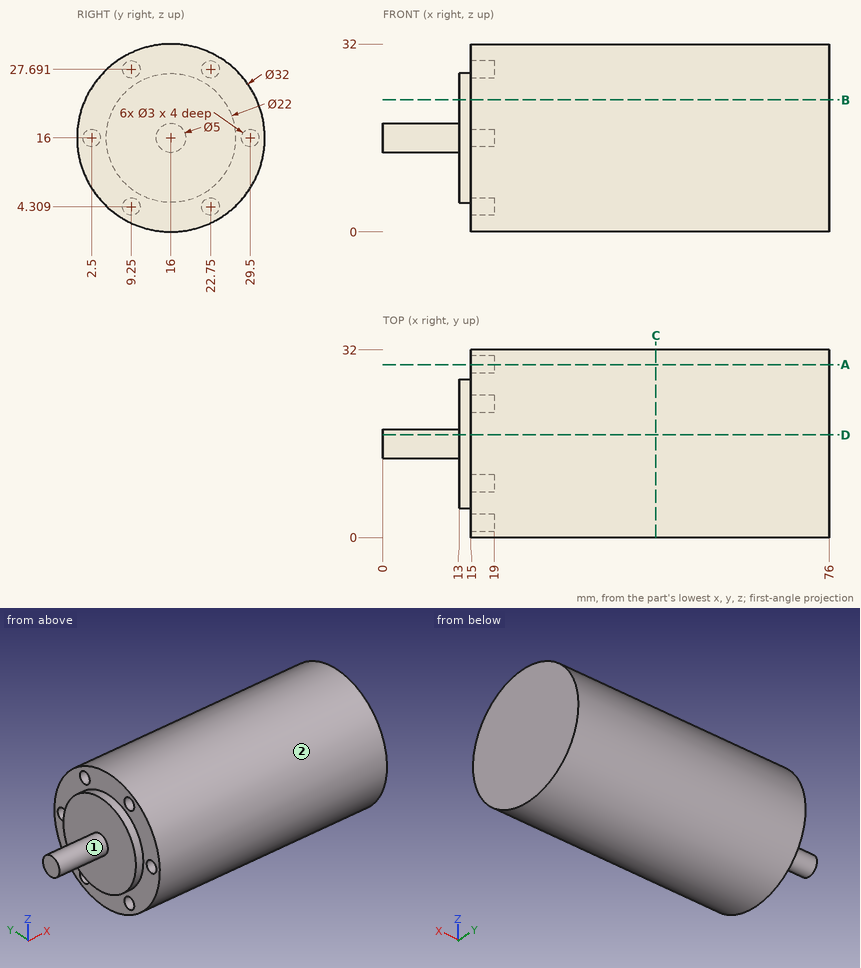
Geometry: see drawing. Coordinates: mm, zero at the bounding-box minimum. A direction names the side the tool comes from. Coordinates: 2 decimals unless noted, no trailing zeros. Order: outer loops, then holes, each group sorted by start corner. A loop starts at its lowest first (then second) coordinate and runs counter-clockwise, first axis right, second up. Notation, with made-up numbers: (3.5, 45.5) - (60.5, 45.5) arc R22 cw to (60.5, 52.5) - close; hole circle Ø2 at (73.25, 60). An arc over 180 degrees is marked (long way). Use one line per item in the form item = value.
1) Section A-A (y = 29.5). Return loops of the section in (x, z).
Solutions:
outline = (15, 7.41) - (76, 7.41) - (76, 24.59) - (15, 24.59) - (15, 17.5) - (19, 17.5) - (19, 14.5) - (15, 14.5) - close
2) Pin query (flat end, axial travel): pin 1 (6 mm diameter, centred on x = 58.5, y = 6.5, fed in from -Z); pin 2 (0.9 mm diameter, centred on y = 3, z = 15.5, fed in from -X); pin 3 (4 mm diameter, centred on y = 7.5, z = 8, fed in from -X). Return the tip coordinate at first contact, or that it passes through.
Solutions:
pin_1 = 1.38
pin_2 = 19
pin_3 = 13
3) Section B-B (z = 22.5). Return loops of the section in (x, y).
Solutions:
outline = (13, 7.13) - (15, 7.13) - (15, 1.38) - (76, 1.38) - (76, 30.62) - (15, 30.62) - (15, 24.87) - (13, 24.87) - close
4) Set-up query: the marked faces 1 and 2. Return all of +Z, -Z, +X, -X, +Y, -Y with unobstructed straight access to the full face (end or side cutting, diameter ignored); none if empty.
Solutions:
face_1 = -X
face_2 = +X, -X
5) Section C-C (x = 46.5). Return loops of the section in (y, z), then the cut area to 3 significant figures.
Solutions:
outline = circle Ø32 at (16, 16)
area = 804 mm^2
6) Ray query, L1, parallel to Y at x = 16.8, z = 16; L2, parallel to Z at x = 15.5, y = 21.5 (1 decimal); L3, parallel to X at y = 8.5, z = 22.5. Return the intervals inside material, ascending.
Solutions:
L1 = 0 to 1, 4 to 28, 31 to 32
L2 = 1 to 3.5, 5.1 to 26.9, 28.5 to 31
L3 = 13 to 76
7) Section D-D (y = 17.5). Return loops of the section in (x, z).
Solutions:
outline = (0, 14) - (13, 14) - (13, 5.1) - (15, 5.1) - (15, 0.07) - (76, 0.07) - (76, 31.93) - (15, 31.93) - (15, 26.9) - (13, 26.9) - (13, 18) - (0, 18) - close
